Geometry: see drawing. Coordinates: mm, zero at the bounding-box minimum. A direction names the side the tool comes from. Coordinates: 2 decimals unless noted, no trailing zeros. Loops run counter-clockwise (first coordinate to the right, second up) from the corner with the lowest first, then second, coordinate; pieces in that order, holes last. Notation, with made-up numbers: (20, 50.5) - (31, 50.5) arc R34 cw to (31, 81.5) - close; hole circle Ø10 at (69, -11). An arc over 180 degrees is marked (long way). Use a Markdown table: item, result. Add a question column.
1. Access query for the marked faces 1, 2 and 3. Directions: +Z, -Z, +X, -X, +Y, -Y. A direction counts if a zero-diameter tool reaches every point of the face in a straight line with its end or side. Return the directions, or none.
2. Contact query for flat-ended pins moving along their axis: P1, Ø5, axis at x = 3, y = 48, coming from the -Z side; P2, Ø4, axis at y = 75, z = 8, coming from the -X side (3 decimals). Output: stop coordinate, or through.
3. Draft query along Z for the marked faces 4, 5, 6 and 7. Return one class per face: released by +Z, released by -Z, zero draft, split by the parting line, or undercut.
4. Section query D-D on x = 30. State how many separate pieces and enclosed holes the cut face has, then the cut area to 3 significant figures.
5. Ray query, L1, parallel to Y at x = 31, z = 38.5; L2, parallel to Z at x = 19.05, y = 38 (1 decimal); L3, parallel to X at y = 65.5, z = 37.5. Return the intervals inside material, ascending. Write a range as [from, to].
6. Section query C-C on z = 41.5. Return the cut outline in (x, y) (1 decimal), then the cut area to 3 significant figures.
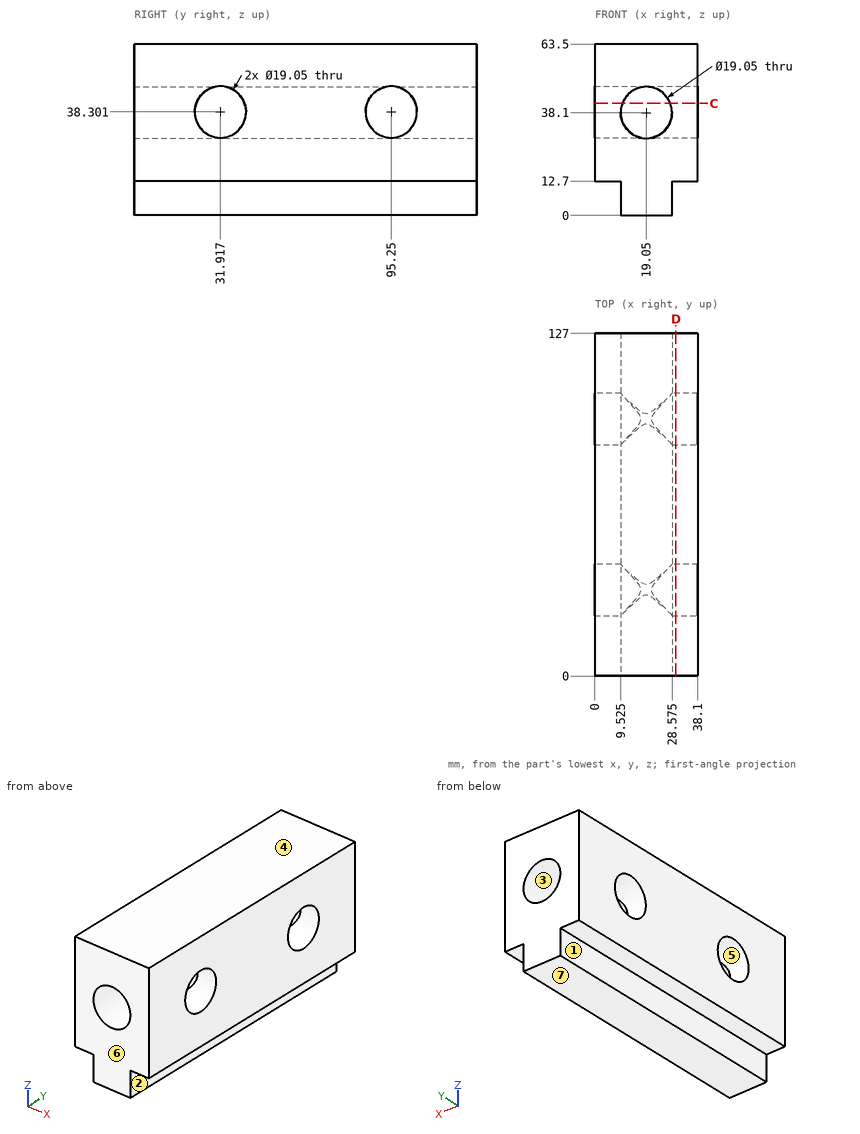
Resolved:
| question | item | result |
|---|---|---|
| 1 | face 1 | -Z, -X, +Y, -Y |
| 1 | face 2 | -Z, +X, +Y, -Y |
| 1 | face 3 | +Y, -Y |
| 2 | P1 | z = 12.7 |
| 2 | P2 | x = 9.525 |
| 3 | face 4 | released by +Z |
| 3 | face 5 | undercut |
| 3 | face 6 | zero draft |
| 3 | face 7 | released by -Z |
| 4 | separate pieces | 1 |
| 4 | enclosed holes | 2 |
| 4 | area | 5,880 mm² |
| 5 | L1 | [0, 22.39], [41.44, 85.73], [104.77, 127] |
| 5 | L2 | [0, 28.6], [47.6, 63.5] |
| 5 | L3 | [0, 9.54], [28.56, 38.1] |
| 6 | outline | (0, 0) - (10.2, 0) - (10.2, 22.9) - (0, 22.9) - close; (0, 40.9) - (10.2, 40.9) - (10.2, 86.3) - (0, 86.3) - close; (0, 104.2) - (10.2, 104.2) - (10.2, 127) - (0, 127) - close; (27.9, 0) - (38.1, 0) - (38.1, 22.9) - (27.9, 22.9) - close; (27.9, 40.9) - (38.1, 40.9) - (38.1, 86.3) - (27.9, 86.3) - close; (27.9, 104.2) - (38.1, 104.2) - (38.1, 127) - (27.9, 127) - close |
| 6 | area | 1,850 mm² |
